Build history of the part. All positions in model axes, mm. Face numbers are marked on the shaded views. A direction names the side the tool comes from. Round coordinates to 2 decimals unless told otherwise and drop trailing zeros. Write each loop counter-clockwise with the first axis right and the second up, starting at its lowest first coordinate (ties: lowest second). Pieces come first, ordered by that corner, then holes.
1) Wall check: probe 1 along Y at (x, z) = (13.75, 5.5); probe 2 along Y at (x, z) = (-1, 1); probe 3 along X at (y, z) = (24, 2). Give the ranges that are in metal, low to high.
2) Saw through at A-A (x = 11.5). Write the cut outline in (y, z).
3) Saw through at C-C (x = -0.5). Write the cut outline in (y, z), plus the area to 3 significant figures.
4) Flat gauge pin, fed straight in: pin 1 (3 mm diameter, centred on x = 11.5, z = 12.5, fed in from +Y). Where does the tip first touch, or does it go through?
5) Which spindle directions (+Z, -Z, +X, -X, +Y, -Y) get a long thin tool onto all of the face, cutting with end or side? Do the marked faces 1 and 2. Say none if no direction does.
6) Saw through at B-B (z = 10.5). Write the cut outline in (x, y), plus the area to 3 significant figures.
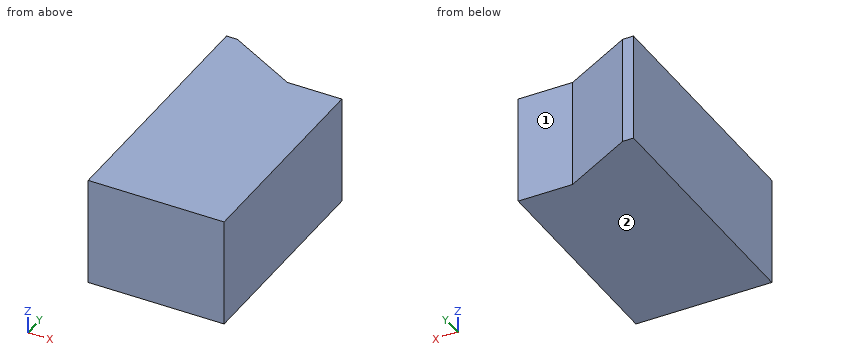
Autodesk Inventor part; units mm, degrees
ref_plane "YZ Plane" through (0, 0, 0) normal (1, 0, 0) x (0, 1, 0)
ref_plane "XZ Plane" through (0, 0, 0) normal (0, 1, 0) x (-1, 0, 0)
ref_plane "XY Plane" through (0, 0, 0) normal (0, 0, 1) x (1, 0, 0)
sketch "Sketch1" plane through (0, 0, 0) normal (0, 0, 1) x (1, 0, 0)
  line L0 (-7.3355, -16.4371) -> (17.6645, -16.4371)
  line L1 (17.6645, -16.4371) -> (17.6645, 23.5629)
  line L2 (-7.3355, -16.4371) -> (-7.3355, 30.5629)
  line L3 (17.6645, 23.5629) -> (7.6645, 23.5629)
  line L4 (7.6645, 23.5629) -> (-5.3355, 30.5629)
  line L5 (-5.3355, 30.5629) -> (-7.3355, 30.5629)
  point P0 (0, 0)
  dimension "d0" = 25
  dimension "d1" = 2
  dimension "d2" = 10
  dimension "d5" = 40
  dimension "d6" = 47
extrude "Extrusion1" add sketch "Sketch1" along normal blind 20
properties part number "3DP_PLA_Pick_up_tray" material "ABS Plastic"
Evaluation:
1. probe 1: y = -16.44 to 23.56
1. probe 2: y = -16.44 to 28.23
1. probe 3: x = -7.34 to 6.85
2. outline: (-16.44, 0) - (23.56, 0) - (23.56, 20) - (-16.44, 20) - close
3. outline: (-16.44, 0) - (27.96, 0) - (27.96, 20) - (-16.44, 20) - close
3. area: 888 mm2
4. pin 1: stops at y = 23.56
5. face 1: +Z, -Z, +X, +Y
5. face 2: -Z, +X, -X, +Y, -Y
6. outline: (-7.34, -16.44) - (17.66, -16.44) - (17.66, 23.56) - (7.66, 23.56) - (-5.34, 30.56) - (-7.34, 30.56) - close
6. area: 1,060 mm2
